Check sheet for the modelled part. Datum: model origin and axes. Units: mm. Face numbers are marked on the shaded views. A direction names the side the tool comes from. Coordinates: 2 decimals unless noted, no trailing zeros. Order: outer loops, then holes, each group sorted by start corner. A loop starts at its lowest first (then second) coordinate and runs counter-clockwise, first axis right, second up.
1. Set-up check for the marked faces 1 and 2: record each of +Z, -Z, +X, -X, +Y, -Y from which the full face is reachable in a straight line by a thin tool's end or side.
2. Cross-section at B-B (z = 17.5). Enter the section's corners in (x, y).
3. Draft check along X on the marked faces 3, 4, 5 and 6. Enter one of: released by +X, released by -X, zero draft, split by the parting line, or undercut.
4. Gauge pin test, flat ends, axial feed: pin 1 Ø3.5 at (x, y) = (-11.5, 11.5) entering from +Z; pin 2 Ø3 at (y, z) = (0.5, 13.5) entering from +X; pin 3 Ø0.8 at (x, y) = (-10.5, 12) entering from +Z. Record the tip position at first contact, or that the pin passes through.
5. Cross-section at A-A (z = 3). Enter the section's corners in (x, y), then the cut area to 3 significant figures.
6. Cross-section at D-D (x = 10.9). Enter the section's corners in (y, z).
7. Cross-section at C-C (y = 3). Enter the section's corners in (x, z).
8. Thickness scan on line 1 (Y direction, x = 10.9, z = 6.75); line 2 (X direction, y = -12, z = 10.75); line 3 (X direction, y = -9.5, z = 15.75). Record the ranges inside material, lowest first.
```python
from build123d import *

# Parameters (mm, degrees)
SKETCH002_R   = 2.2
SKETCH002_R_2 = 1.3
SKETCH002_W   = 3
SKETCH002_H   = 3
PAD_DEPTH     = 7
SKETCH_W      = 31.2
SKETCH_H      = 31.2
SKETCH_W_2    = 28.8
SKETCH_H_2    = 28.8
PAD002_DEPTH  = 18.8
SKETCH003_W   = 3
SKETCH003_H   = 3
PAD003_DEPTH  = 2
PAD001_DEPTH  = 1.2


with BuildPart() as pad:
    # Sketch002 → Pad (new body)
    with BuildSketch(Plane.XY.offset(1.2)):
        with Locations((-10.9, 11.4)):
            Circle(SKETCH002_R)
        with Locations((-10.9, 11.4)):
            Circle(SKETCH002_R_2, mode=Mode.SUBTRACT)
        with Locations((10.9, 11.4)):
            Circle(SKETCH002_R)
        with Locations((10.9, 11.4)):
            Circle(SKETCH002_R_2, mode=Mode.SUBTRACT)
        with Locations((-12.9, -12.9)):
            Rectangle(SKETCH002_W, SKETCH002_H)
    extrude(amount=PAD_DEPTH)


with BuildPart() as pad002:
    # Sketch → Pad002 (new body)
    with BuildSketch(Plane.XY.offset(1.2)):
        Rectangle(SKETCH_W, SKETCH_H)
        Rectangle(SKETCH_W_2, SKETCH_H_2, mode=Mode.SUBTRACT)
    extrude(amount=PAD002_DEPTH)


with BuildPart() as pad003:
    # Sketch003 → Pad003 (new body)
    with BuildSketch(Plane.XY.offset(10)):
        with Locations((-12.9, -12.9)):
            Rectangle(SKETCH003_W, SKETCH003_H)
    extrude(amount=PAD003_DEPTH)


with BuildPart() as fusion:
    # Sketch001 → Pad001 (new body)
    with BuildSketch(Plane.XY):
        with BuildLine():
            Line((-15.6, 15.6), (15.6, 15.6))
            Line((15.6, 15.6), (15.6, -10.6))
            Line((15.6, -10.6), (17.6, -10.60001))
            ThreePointArc((17.6, -15.6), (20.099979, -13.100005), (17.6, -10.60001))
            Line((15.6, -15.6), (17.6, -15.6))
            Line((15.6, -15.6), (-15.6, -15.6))
            Line((-15.6, -15.6), (-15.6, 10.6))
            Line((-17.6, 10.6), (-15.6, 10.6))
            ThreePointArc((-17.6, 15.6), (-20.099999, 13.1), (-17.6, 10.6))
            Line((-17.6, 15.6), (-15.6, 15.6))
        make_face()
    extrude(amount=PAD001_DEPTH)

    # Fusion: union Pad, Pad002, Pad003
    add(pad.part)
    add(pad002.part)
    add(pad003.part)


solid = fusion.part
```
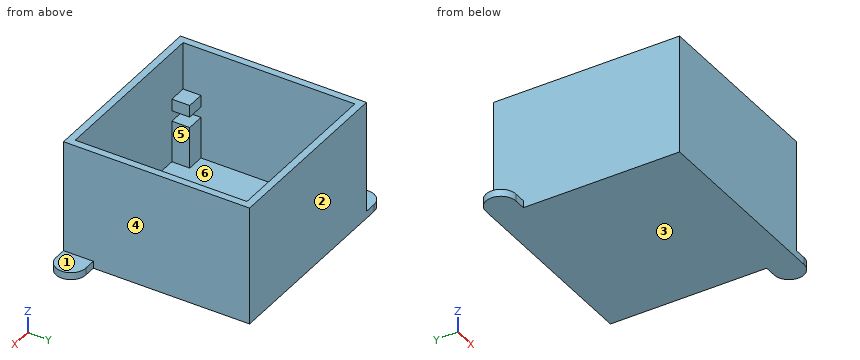
Data:
1. face 1: +Z, +X, +Y, -Y
1. face 2: +Z, -Z, +X, -X, +Y
2. outline: (-15.6, -15.6) - (15.6, -15.6) - (15.6, 15.6) - (-15.6, 15.6) - close; hole (-14.4, -14.4) - (14.4, -14.4) - (14.4, 14.4) - (-14.4, 14.4) - close
3. face 3: zero draft
3. face 4: released by +X
3. face 5: undercut
3. face 6: undercut
4. pin 1: stops at z = 8.2
4. pin 2: stops at x = 15.6
4. pin 3: stops at z = 1.2
5. outline: (-15.6, -15.6) - (15.6, -15.6) - (15.6, 15.6) - (-15.6, 15.6) - close; circle Ø4.4 at (-10.9, 11.4); circle Ø4.4 at (10.9, 11.4); hole (-14.4, -11.4) - (-11.4, -11.4) - (-11.4, -14.4) - (14.4, -14.4) - (14.4, 14.4) - (-14.4, 14.4) - close; hole circle Ø2.6 at (-10.9, 11.4); hole circle Ø2.6 at (10.9, 11.4)
5. area: 173 mm2
6. outline: (-15.6, 0) - (15.6, 0) - (15.6, 20) - (14.4, 20) - (14.4, 1.2) - (13.6, 1.2) - (13.6, 8.2) - (12.7, 8.2) - (12.7, 1.2) - (10.1, 1.2) - (10.1, 8.2) - (9.2, 8.2) - (9.2, 1.2) - (-14.4, 1.2) - (-14.4, 20) - (-15.6, 20) - close
7. outline: (-15.6, 0) - (15.6, 0) - (15.6, 20) - (14.4, 20) - (14.4, 1.2) - (-14.4, 1.2) - (-14.4, 20) - (-15.6, 20) - close
8. line 1: y = -15.6 to -14.4, 9.2 to 10.1, 12.7 to 13.6, 14.4 to 15.6
8. line 2: x = -15.6 to -11.4, 14.4 to 15.6
8. line 3: x = -15.6 to -14.4, 14.4 to 15.6
